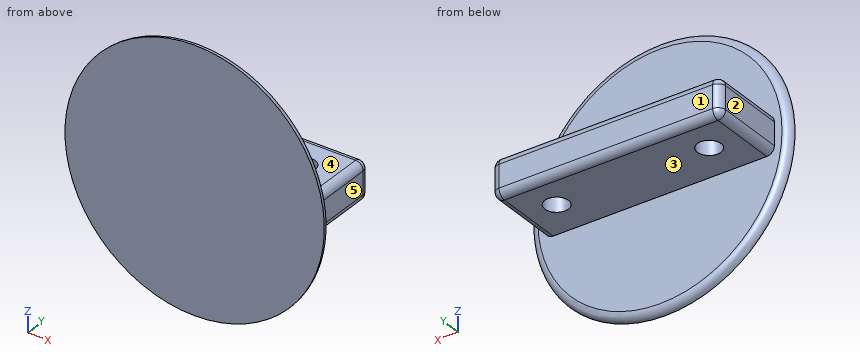
from build123d import *

# Parameters (mm, degrees)
SKETCH1_W                      = 76.2
SKETCH1_H                      = 25.4
BOSS_EXTRUDE1_DEPTH            = 6.35
FILLET1_R                      = 2.54
F_97_0_31_DIAMETER_HOLE1_D     = 7.874
F_97_0_31_DIAMETER_HOLE1_DEPTH = 25.4
F_97_0_31_DIAMETER_HOLE1_TIP   = 2.365588257
SKETCH4_R                      = 43.18
BOSS_EXTRUDE2_DEPTH            = 2.54
FILLET2_R                      = 2.54


with BuildPart() as part:
    # Sketch1 → Boss-Extrude1 (new, symmetric)
    with BuildSketch(Plane.XY):
        Rectangle(SKETCH1_W, SKETCH1_H)
    extrude(amount=BOSS_EXTRUDE1_DEPTH, both=True)

    # Fillet1
    fillet1_edges = [part.edges().sort_by_distance(p)[0] for p in [
        (-38.1, 0, 6.35),
        (38.1, 0, 6.35),
        (-38.1, 0, -6.35),
        (0, 12.7, -6.35),
        (38.1, 0, -6.35),
        (-38.1, 12.7, 0),
        (38.1, 12.7, 0),
        (0, 12.7, 6.35),
    ]]
    fillet(fillet1_edges, radius=FILLET1_R)

    # #97 (0.31) Diameter Hole1
    with Locations(Plane.XY.offset(6.35)):
        with Locations((25.4, 0), (-25.4, 0)):
            Hole(F_97_0_31_DIAMETER_HOLE1_D / 2, depth=F_97_0_31_DIAMETER_HOLE1_DEPTH)
            with Locations((0, 0, -(F_97_0_31_DIAMETER_HOLE1_DEPTH + F_97_0_31_DIAMETER_HOLE1_TIP / 2))):  # 118° drill point
                Cone(0, F_97_0_31_DIAMETER_HOLE1_D / 2, F_97_0_31_DIAMETER_HOLE1_TIP, mode=Mode.SUBTRACT)

    # Sketch4 → Boss-Extrude2 (add)
    with BuildSketch(Plane.XZ.offset(12.7)):
        with Locations(Location((0, 0, 0), (0, 0, 270))):
            Circle(SKETCH4_R)
    extrude(amount=BOSS_EXTRUDE2_DEPTH)

    # Fillet2
    fillet2_edges = [part.edges().sort_by_distance(p)[0] for p in [
        (0, -12.7, 43.18),
    ]]
    fillet(fillet2_edges, radius=FILLET2_R - 0.0001)  # a hair under: the kernel refuses the full size


solid = part.part
The listing builds one solid part. Answer for the finished solid, in the listing's coordinates (mm). Face numbers are marked on the shaded views. A direction names the side the tool comes from. Give positions to 0.01 mm unless a question says otherwise; leave off trailing zeros. Write each loop counter-clockwise with the first axis right and the second up, starting at its lowest first coordinate (ties: lowest second). Pieces come first, ordered by that corner, then holes. Notation, with made-up numbers: (-25.75, 18.25) - (31.25, 18.25) arc R29 cw to (31.25, 41.25) - close; hole circle Ø11 at (49, -4). An arc over 180 degrees is marked (long way). Use a Markdown table: item, result.
1. Section A-A on y = 0 is taken. Write down the section's boundary in (x, z), plus the area to 3 significant figures.
Values follow:
| item | result |
|---|---|
| outline | (-38.1, -3.81) arc R2.54 ccw to (-35.56, -6.35) - (-29.34, -6.35) - (-29.34, 6.35) - (-35.56, 6.35) arc R2.54 ccw to (-38.1, 3.81) - close; (-21.46, -6.35) - (21.46, -6.35) - (21.46, 6.35) - (-21.46, 6.35) - close; (29.34, -6.35) - (35.56, -6.35) arc R2.54 ccw to (38.1, -3.81) - (38.1, 3.81) arc R2.54 ccw to (35.56, 6.35) - (29.34, 6.35) - close |
| area | 762 mm² |
2. Each of these flat-tipped pins is pushed along its axis until it touches: P1, Ø1, axis at x = 12, y = -1.5, coming from the -Z side; P2, Ø1.5, axis at x = 22, y = -3, coming from the +Z side; P3, Ø2.5, axis at y = -6.5, z = -1, coming from the +X side. Where does it stop, or does it pass through?
Values follow:
| item | result |
|---|---|
| P1 | stops at z = -6.35 |
| P2 | stops at z = 6.35 |
| P3 | stops at x = 38.1 |
3. Find the intervals of material crossed by probe 1 along Y at (x, z) = (25, 2); probe 2 along X at (y, z) = (7.75, -4); probe 3 along Y at (x, z) = (23, -17.5), in increasing order. Write a range as from..to.
Values follow:
| item | result |
|---|---|
| probe 1 | y = -15.24..-3.92, 3.92..12.7 |
| probe 2 | x = -38.09..38.09 |
| probe 3 | y = -15.24..-12.7 |
4. Section D-D on y = -11.5 is taken. Write down the section's boundary in (x, z).
Values follow:
| item | result |
|---|---|
| outline | (-38.1, -3.81) arc R2.54 ccw to (-35.56, -6.35) - (35.56, -6.35) arc R2.54 ccw to (38.1, -3.81) - (38.1, 3.81) arc R2.54 ccw to (35.56, 6.35) - (-35.56, 6.35) arc R2.54 ccw to (-38.1, 3.81) - close |
5. A tool of negligible diameter and unlimited length cuts with its end or side. For the marked faces 1, 2, 3, 4 and 5, from which of +Z, -Z, +X, -X, +Y, -Y can it reach the whole face along a straight path? Write none if from no direction.
Values follow:
| item | result |
|---|---|
| face 1 | +Z, -Z, +X, -X, +Y |
| face 2 | +Z, -Z, -X, +Y |
| face 3 | -Z, +X, -X, +Y |
| face 4 | +Z, +X, -X, +Y |
| face 5 | +Z, -Z, +X, +Y |
6. Section B-B on z = 0 is taken. Count the separate pieces of the cut face and the enclosed holes in it, plus the area to 3 significant figures.
Values follow:
| item | result |
|---|---|
| separate pieces | 1 |
| enclosed holes | 2 |
| area | 2,050 mm² |
